The figure shows three views and two pictorial views of one solid part (mm, origin at its lowest corner). Answer the questions. A direction names the side the tool comes from. Give positions to 0.01 mm unless a question says otherwise; leave off trailing zeros. Order: outer loops, then holes, each group sorted by start corner. A loop starts at its lowest first (then second) coordinate and runs counter-clockwise, first axis right, second up. Notation, with made-up numbers: (12.25, 27.5) - (58.25, 27.5) arc R14 ccw to (58.25, 36.5) - close; hole circle Ø2 at (-21, -1). An arc over 180 degrees is marked (long way). Write item = value, one per line.
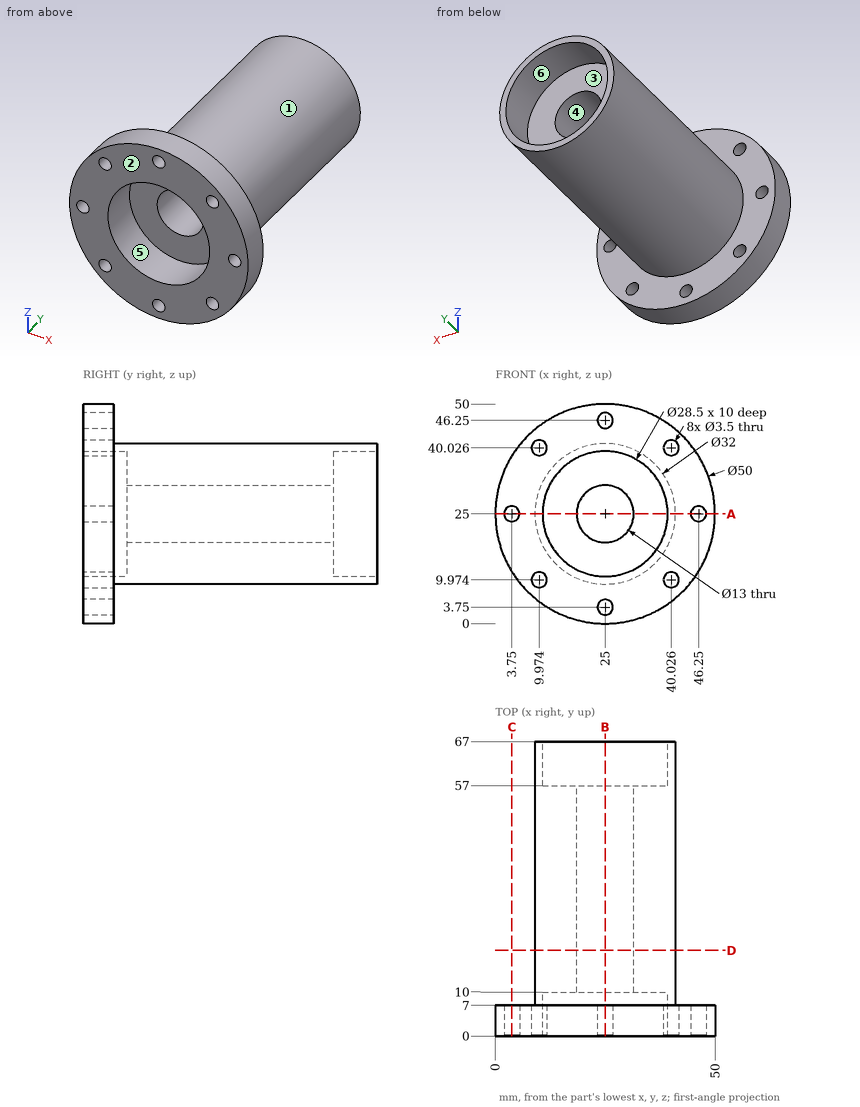
1. Section B-B (x = 25) is taken. Determine the outline of the cut face in (y, z).
Recorded:
outline = (0, 0) - (7, 0) - (7, 2) - (0, 2) - close; (0, 5.5) - (7, 5.5) - (7, 9) - (67, 9) - (67, 10.75) - (57, 10.75) - (57, 18.5) - (10, 18.5) - (10, 10.75) - (0, 10.75) - close; (0, 39.25) - (10, 39.25) - (10, 31.5) - (57, 31.5) - (57, 39.25) - (67, 39.25) - (67, 41) - (7, 41) - (7, 44.5) - (0, 44.5) - close; (0, 48) - (7, 48) - (7, 50) - (0, 50) - close
2. Section D-D (y = 19.5) is taken. Determine the outline of the cut face in (x, z).
Recorded:
outline = circle Ø32 at (25, 25); hole circle Ø13 at (25, 25)
3. Flat-ended cylindrical pins translate along their axes: pin 1 (3 mm diameter, centred on x = 9.97, z = 9.97, fed in from +Y); pin 2 (1 mm diameter, centred on x = 15, y = 45, fed in from -Z); pin 3 (10 mm diameter, centred on y = 13, z = 35.5, fed in from +X) (3 decimals); pin 4 (10 mm diameter, centred on y = 39, z = 30, fed in from +X). Find the tip coordinate at first contact, or state that the pin passes through.
Recorded:
pin_1 = through
pin_2 = 12.13
pin_3 = 40.025
pin_4 = 41
4. Determine the mould class of the marked faces 1, 2 and 3 for opening direction X: +X half, -X half, draft (parallel to the pull), parting line (faces both ways), or undercut.
Recorded:
face_1 = parting line
face_2 = draft
face_3 = undercut
5. Straight lines are drawn through the part: L1, parallel to X at y = 6.5, z = 25; L2, parallel to X at y = 41, z = 24.5; L3, parallel to X at y = 63, z = 25. For each, find the intervals that lie inside material, in ascending order. Write a range as [from, to].
Recorded:
L1 = [0, 2], [5.5, 10.75], [39.25, 44.5], [48, 50]
L2 = [9.01, 18.52], [31.48, 40.99]
L3 = [9, 10.75], [39.25, 41]
6. For the marked faces 4, 5 and 6, determine the directions among +Z, -Z, +X, -X, +Y, -Y from which every point of the face is accessible in a straight line to the end or side of a thin tool.
Recorded:
face_4 = +Y, -Y
face_5 = -Y
face_6 = +Y
7. Section C-C (x = 3.75) is taken. Determine the outline of the cut face in (y, z).
Recorded:
outline = (0, 11.83) - (7, 11.83) - (7, 23.25) - (0, 23.25) - close; (0, 26.75) - (7, 26.75) - (7, 38.17) - (0, 38.17) - close
8. Section A-A (z = 25) is taken. Determine the outline of the cut face in (x, y).
Recorded:
outline = (0, 0) - (2, 0) - (2, 7) - (0, 7) - close; (5.5, 0) - (10.75, 0) - (10.75, 10) - (18.5, 10) - (18.5, 57) - (10.75, 57) - (10.75, 67) - (9, 67) - (9, 7) - (5.5, 7) - close; (31.5, 10) - (39.25, 10) - (39.25, 0) - (44.5, 0) - (44.5, 7) - (41, 7) - (41, 67) - (39.25, 67) - (39.25, 57) - (31.5, 57) - close; (48, 0) - (50, 0) - (50, 7) - (48, 7) - close
